Geometry: see drawing. Coordinates: mm, zero at the bounding-box minimum. A direction names the side the tool comes from. Round coordinates to 2 decimals unless told otherwise and drop trailing zeros. Loops run counter-clockwise (first coordinate to the right, second up) from the corner with the lowest first, then second, coordinate; pieces in that order, holes last. Notation, with made-up numbers: (64.25, 54.25) -> (112.25, 54.25) arc R22 ccw to (112.25, 92.25) -> close; hole circle Ø11 at (-3.5, 6.5). An arc over 180 degrees is marked (long way). Write item = value, one per line.
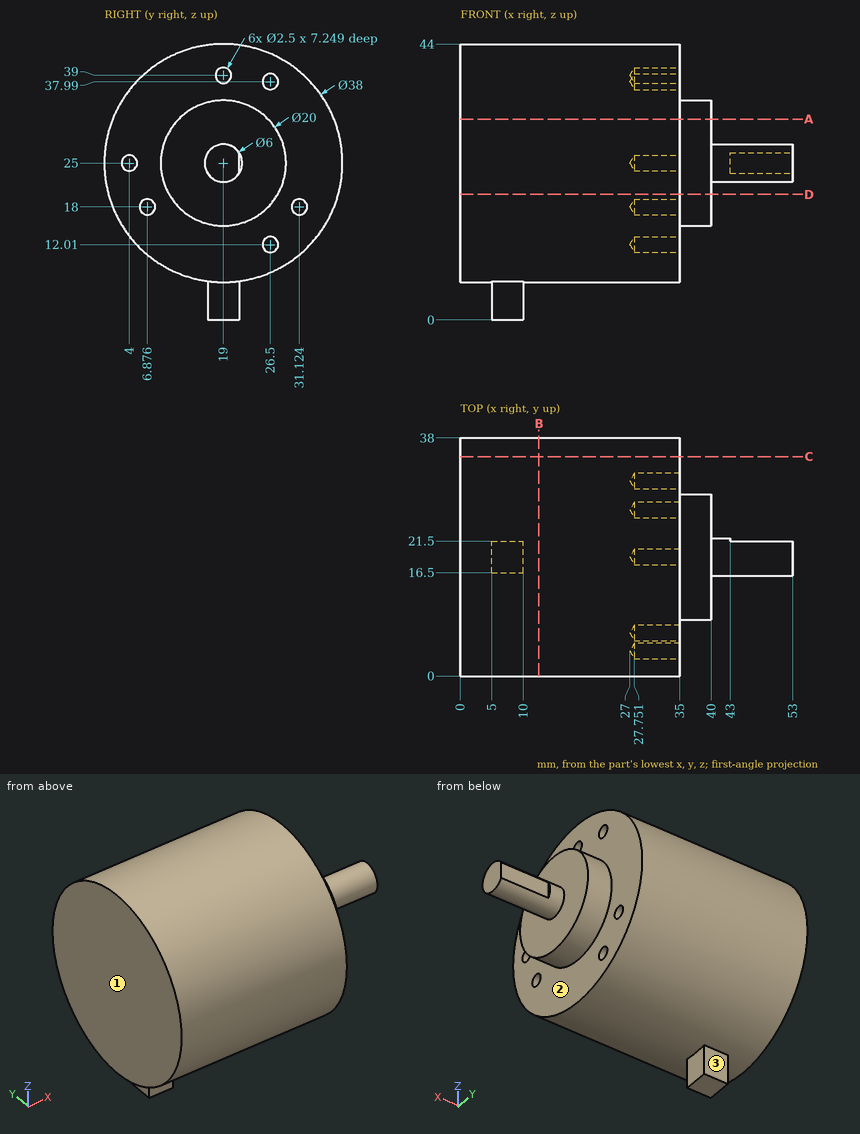
1. Contact query for flat-ended pins moving along their axis: pin 1 Ø1.7 at (x, z) = (50, 24.5) entering from +Y; pin 2 Ø10 at (y, z) = (11.5, 31) entering from +X; pin 3 Ø2 at (x, z) = (31.5, 20) entering from +Y; pin 4 Ø3 at (x, y) = (43.5, 24.5) entering from -Z. Output: stop coordinate, or through.
Evaluation:
pin_1 = 21.5
pin_2 = 40
pin_3 = 37.57
pin_4 = through
2. Section query A-A (z = 32). Return the cut outline in (x, y).
Evaluation:
outline = (0, 1.34) -> (35, 1.34) -> (35, 11.86) -> (40, 11.86) -> (40, 26.14) -> (35, 26.14) -> (35, 36.66) -> (0, 36.66) -> close
3. Section query C-C (y = 35). Return the cut outline in (x, z), then the cut area to 3 significant figures.
Evaluation:
outline = (0, 14.75) -> (35, 14.75) -> (35, 35.25) -> (0, 35.25) -> close
area = 717 mm²
4. Section query D-D (z = 20). Return the cut outline in (x, y), then the cut area to 3 significant figures.
Evaluation:
outline = (0, 0.67) -> (35, 0.67) -> (35, 10.34) -> (40, 10.34) -> (40, 27.66) -> (35, 27.66) -> (35, 37.33) -> (0, 37.33) -> close
area = 1,370 mm²
5. Line query: probe 1 along Z at (x, y) = (50, 16.5); probe 2 along X at (y, z) = (5, 31); probe 3 along X at (y, z) = (14.5, 22.5). Output: solid intervals per line, ascending. Write a range as from..to.
Evaluation:
probe_1 = 23.34..26.66
probe_2 = 0..35
probe_3 = 0..40
6. Section query B-B (x = 12.5). Return the cut outline in (y, z).
Evaluation:
outline = circle Ø38 at (19, 25)
7. Set-up query: the marked faces 1, 2 and 3. Return all of +Z, -Z, +X, -X, +Y, -Y with unobstructed straight access to the full face (end or side cutting, diameter ignored); none if empty.
Evaluation:
face_1 = +Z, -Z, -X, +Y, -Y
face_2 = +X
face_3 = -Z, +X, -X, +Y
